Can you work these out from the model? Positions are in its coordinate system, mm. A direction names the side the tool comes from. Round coordinates to 2 decimals unless told otherwise and drop trailing zeros. Write each loop counter-clockwise with the first axis right and the second up, starting at its lowest first coordinate (ties: lowest second). Pieces come first, ordered by that corner, then holes. Notation, with made-up numbers: M -2.5,87 L 8.5,87 A17 cw 8.5,102 Z; hole C -5,22.25 d7. An arc over 180 degrees is marked long. Answer as a JSON object with one key per item and string values. Group by question number.
1) Suppose I cut it at D-D, the plane x = 17.5. Write out the boundary of the cut face in (y, z) (3 decimals), and give its area (3 significant figures).
2) I'm going to push flat-ended pins straight in: pin 1 Ø2 at (x, y) = (1.5, -13.5) entering from +Z; pin 2 Ø10 at (x, z) = (20.5, 43.5) entering from +Y (3 decimals); pin 3 Ø7.5 at (y, z) = (2.5, 35.5) entering from -X; pin 4 Ø19.5 at (x, y) = (-25.4, 0) entering from +Z. Where does each tip first touch, or does it pass through?
3) Suppose I cut it at C-C, the plane z = 21.5. Write out the boundary of the cut face in (x, y) (3 decimals), and give its area (3 significant figures).
4) Suppose I cut it at A-A, the plane y = 0. Write out the boundary of the cut face in (x, z) (3 decimals), and give its area (3 significant figures).
5) On a 3-axis mill with a long thin cutter (end or side, diameter ignored), from which of +Z, -Z, +X, -X, +Y, -Y can I reach the whole of each face in a straight line? I mean faces 1 (the flat face through (-11, 0, 25.4)), 2 (the flat face through (5, -22.225, 19)), 3 (the flat face through (19, 16, 38.1)). Say none if no direction works.
6) Suppose I cut it at B-B, the plane x = -31.5. Write out the boundary of the cut face in (y, z), and give its area (3 significant figures).
7) Please list where these lines run through material, in increasing order: L1, parallel to Y at x = -25, z = 9 (3 decimals); L2, parallel to Z at x = -1, y = 18; L3, parallel to X at y = -18.5, z = 33.5. Write a range as [from, to].
8) If we mould it in two halves opening along Y, with no side actions, what happens to faces 4 (the flat face through (25.4, 0, 25)), 5 (the cylindrical face through (-33.356, 7.296, 12.878)), 6 (the flat face through (19, 9.525, 45)), 7 (the cylindrical face through (-47.62, 0.49, 12.52))? For each: +Y half, -Y half, draft (parallel to the pull), parting line (faces both ways), or undercut.
from build123d import *

# Parameters (mm, degrees)
F0_W     = 50.8
F0_H     = 44.45
F1_DEPTH = 25.4
F2_R     = 22.225
F3_DEPTH = 25.4
F4_R     = 10.795
F5_DEPTH = 25.401
F6_W     = 12.7
F6_H     = 44.45
F7_DEPTH = 25.4
F8_W     = 12.7
F8_H     = 12.7
F9_DEPTH = 12.7


with BuildPart() as f1:
    # F0 (on Top) → F1 (new body)
    with BuildSketch(Plane.XY):
        Rectangle(F0_W, F0_H)
    extrude(amount=F1_DEPTH)

    # F2 (on Top) → F3 (join)
    with BuildSketch(Plane.XY):
        with Locations((-25.4, 0)):
            Circle(F2_R)
    extrude(amount=F3_DEPTH)

    # F4 (on face) → F5 (cut, through all)
    with BuildSketch(Plane.XY.offset(25.4)):
        with Locations((-25.4, 0)):
            Circle(F4_R)
    extrude(amount=-F5_DEPTH, mode=Mode.SUBTRACT)

    # F6 (on face) → F7 (join)
    with BuildSketch(Plane.XY.offset(25.4)):
        with Locations((19.05, 0)):
            Rectangle(F6_W, F6_H)
    extrude(amount=F7_DEPTH)

    # F8 (on face) → F9 (cut)
    with BuildSketch(Plane.XY.offset(50.8)):
        with Locations((19.05, 15.875)):
            Rectangle(F8_W, F8_H)
    extrude(amount=-F9_DEPTH, mode=Mode.SUBTRACT)


solid = f1.part
Results:
{
 "1": {"outline": "M -22.225,0 L 22.225,0 L 22.225,38.1 L 9.525,38.1 L 9.525,50.8 L -22.225,50.8 Z", "area": "2,100 mm^2"},
 "2": {"pin 1": "z = 25.4", "pin 2": "y = 9.525", "pin 3": "x = 12.7", "pin 4": "through"},
 "3": {"outline": "M -25.4,-22.225 L 25.4,-22.225 L 25.4,22.225 L -25.4,22.225 A22.225 ccw Z; hole C -25.4,0 d21.59", "area": "2,670 mm^2"},
 "4": {"outline": "M -47.625,0 L -36.195,0 L -36.195,25.4 L -47.625,25.4 Z; M -14.605,0 L 25.4,0 L 25.4,50.8 L 12.7,50.8 L 12.7,25.4 L -14.605,25.4 Z", "area": "1,630 mm^2"},
 "5": {"face 1": "+Z, -X, +Y, -Y", "face 2": "+Z, -Z, +X, -X, -Y", "face 3": "+Z, +X, -X, +Y"},
 "6": {"outline": "M -21.37,0 L -8.91,0 L -8.91,25.4 L -21.37,25.4 Z; M 8.91,0 L 21.37,0 L 21.37,25.4 L 8.91,25.4 Z", "area": "633 mm^2"},
 "7": {"L1": "[-22.225, -10.788], [10.788, 22.225]", "L2": "[0, 25.4]", "L3": "[12.7, 25.4]"},
 "8": {"face 4": "draft", "face 5": "undercut", "face 6": "+Y half", "face 7": "parting line"}
}
